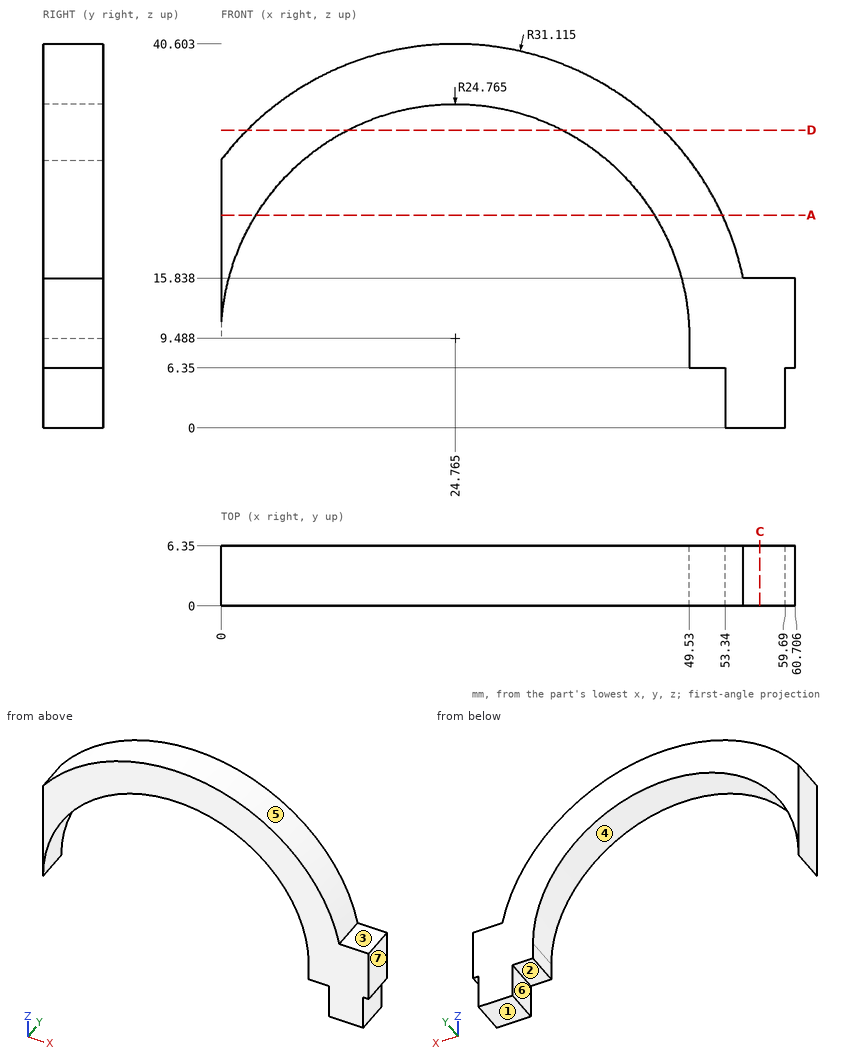
Source: three-view drawing plus pictorial views. Frame: mm from the lowest corner of the part. A direction names the side the tool comes from. Coordinates: 2 decimals unless noted, no trailing zeros. Order: outer loops, then holes, each group sorted by start corner. A loop starts at its lowest first (then second) coordinate and runs counter-clockwise, first axis right, second up. Notation, with made-up numbers: M 83,62.25 L 102,62.25 A18 cw 102,72.25 Z; hole C 1,77.25 d7. An arc over 180 degrees is marked long. Answer in a Markdown table with one row per item.
(1) Section query D-D, the plane z = 31.5. Output: boundary loops of the cut face in (x, y).
Numbers:
| item | result |
|---|---|
| outline | M 2.77,0 L 13.42,0 L 13.42,6.35 L 2.77,6.35 Z; M 36.11,0 L 46.76,0 L 46.76,6.35 L 36.11,6.35 Z |
(2) Contact query for flat-ended pins moving along their axis: pin 1 Ø1.6 at (y, z) = (4, 8) entering from -X; pin 2 Ø2.5 at (x, y) = (57.5, 4) entering from +Z; pin 3 Ø1.5 at (x, y) = (53.5, 1.5) entering from +Z. Output: stop coordinate, or through.
Numbers:
| item | result |
|---|---|
| pin 1 | stops at x = 49.53 |
| pin 2 | stops at z = 15.84 |
| pin 3 | stops at z = 23.09 |
(3) Draft query along X for the marked faces 4, 5, 6 and 7. Return one class per face: pulls with the +X half, pulls with the -X half, needs draft (parallel to the pull), parting line crosses it, or undercut.
Numbers:
| item | result |
|---|---|
| face 4 | undercut |
| face 5 | parting line crosses it |
| face 6 | pulls with the -X half |
| face 7 | pulls with the +X half |
(4) Access query for the marked faces 1, 2 and 3. Directions: +Z, -Z, +X, -X, +Y, -Y. A direction counts if a zero-diameter tool reaches every point of the face in a straight line with its end or side. Return the directions, or none.
Numbers:
| item | result |
|---|---|
| face 1 | -Z, +X, -X, +Y, -Y |
| face 2 | -Z, -X, +Y, -Y |
| face 3 | +Z, +X, +Y, -Y |
(5) Material intervals for line 1 (X direction, y = 3, z = 17.5); line 2 (Z direction, x = 58, y = 3.75); line 3 (X direction, y = 1, z = 24), sorted ascending. Write a range as [from, to].
Numbers:
| item | result |
|---|---|
| line 1 | x = [0, 1.33], [48.2, 54.83] |
| line 2 | z = [0, 15.84] |
| line 3 | x = [0, 4.7], [44.83, 52.29] |
(6) Section query C-C, the plane x = 57. Output: boundary loops of the cut face in (y, z).
Numbers:
| item | result |
|---|---|
| outline | M 0,0 L 6.35,0 L 6.35,15.84 L 0,15.84 Z |
(7) Section query A-A, the plane z = 22.5. Output: boundary loops of the cut face in (x, y).
Numbers:
| item | result |
|---|---|
| outline | M 0,0 L 3.69,0 L 3.69,6.35 L 0,6.35 Z; M 45.84,0 L 53.03,0 L 53.03,6.35 L 45.84,6.35 Z |
